from build123d import *

# Parameters (mm, degrees)
SKETCH1_R               = 32
BOSS_EXTRUDE1_DEPTH     = 15
SKETCH2_R               = 7
SKETCH2_R_2             = 6.446135322
BOSS_EXTRUDE2_DEPTH     = 15
SKETCH3_R               = 5.5
BOSS_EXTRUDE3_DEPTH     = 79
CUT_EXTRUDE1_DEPTH      = 79
CUT_EXTRUDE1_DEPTH_BACK = 79


with BuildPart() as part:
    # Sketch1 → Boss-Extrude1 (new body)
    with BuildSketch(Plane(origin=(0, 0, 0), x_dir=(1, 0, 0), z_dir=(0, 1, 0))):
        Circle(SKETCH1_R)
    extrude(amount=BOSS_EXTRUDE1_DEPTH)

    # Sketch2 → Boss-Extrude2 (add)
    with BuildSketch(Plane(origin=(0, 15, 0), x_dir=(1, 0, 0), z_dir=(0, 1, 0))):
        with Locations((25, 0)):
            Circle(SKETCH2_R)
        with Locations((-13, 22)):
            Circle(SKETCH2_R_2)
        with Locations((-13, -22)):
            Circle(SKETCH2_R_2)
    extrude(amount=BOSS_EXTRUDE2_DEPTH)

    # Sketch3 → Boss-Extrude3 (add)
    with BuildSketch(Plane(origin=(0, 15, 0), x_dir=(1, 0, 0), z_dir=(0, 1, 0))):
        Circle(SKETCH3_R)
    extrude(amount=BOSS_EXTRUDE3_DEPTH)

    # Sketch4 → Cut-Extrude1 (cut, two sides)
    with BuildSketch(Plane(origin=(0, 0, 0), x_dir=(0, 0, -1), z_dir=(1, 0, 0))) as cut_extrude1_sk:
        Polygon((-4.5, 84), (-8.757640736, 84), (-8.757640736, 94), (-4.5, 94), (-4, 94), (-4, 84), align=None)
    extrude(amount=CUT_EXTRUDE1_DEPTH, mode=Mode.SUBTRACT)
    extrude(cut_extrude1_sk.sketch, amount=-CUT_EXTRUDE1_DEPTH_BACK, mode=Mode.SUBTRACT)


solid = part.part
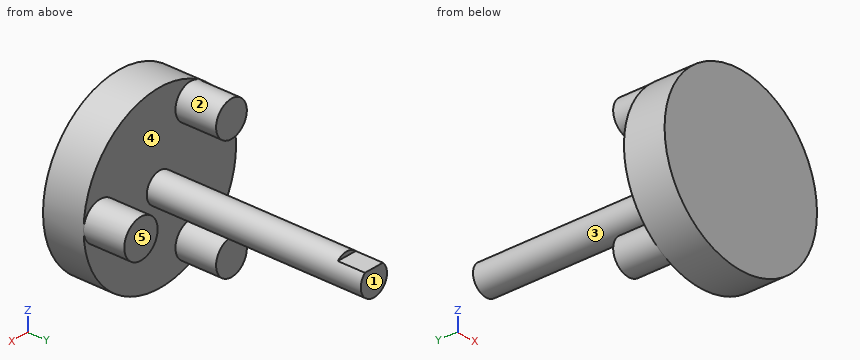
Geometry: final body of the model. Coordinates: model frame, mm. Face numbers are marked on the shaded views. A direction names the side the tool comes from. Round coordinates to 2 decimals unless told otherwise and drop trailing zeros. Order: outer loops, then holes, each group sorted by start corner. A loop starts at its lowest first (then second) coordinate and runs counter-clockwise, first axis right, second up. Notation, with made-up numbers: (51, -7.75) - (79, -7.75) arc R29 cw to (79, 21.25) - close; hole circle Ø1 at (-16, -12.5). An arc over 180 degrees is marked (long way). Write each question's results on one line, items separated by ' | '.
Item 1: Section C-C, the plane y = 45. Return the cut outline in (x, z).
Completed:
outline: circle Ø11 at (0, 0)
Item 2: Mould query, pull axis Z, two halves, no side actions, for the marked faces 3, 4 and 5. Classes: pulls with the +Z half, pulls with the -Z half, needs draft (parallel to the pull), parting line crosses it, or undercut.
Completed:
face 3: parting line crosses it | face 4: undercut | face 5: needs draft
Item 3: Section A-A, the plane x = 0. Return the cut outline in (y, z), and give its area (3 significant figures).
Completed:
outline: (0, -32) - (15, -32) - (15, -5.5) - (94, -5.5) - (94, 4) - (84, 4) - (84, 5.5) - (15, 5.5) - (15, 32) - (0, 32) - close | area: 1,810 mm^2
Item 4: Material intervals for line 1 along Y through (x, z) = (-6, 26); line 2 along Z through (x, y) = (23, 21); line 3 along Z through (x, y) = (-3.5, 89), sorted ascending. Write a range as [from, to].
Completed:
line 1: [0, 15] | line 2: [-6.71, 6.71] | line 3: [-4.24, 4]
Item 5: Section B-B, the plane z = -4. Return the cut outline in (x, y), and give its area (3 significant figures).
Completed:
outline: (-31.75, 0) - (31.75, 0) - (31.75, 15) - (30.74, 15) - (30.74, 30) - (19.26, 30) - (19.26, 15) - (3.77, 15) - (3.77, 94) - (-3.77, 94) - (-3.77, 15) - (-31.75, 15) - close | area: 1,720 mm^2
Item 6: Section D-D, the plane z = -25. Return the cut outline in (x, y).
Completed:
outline: (-19.97, 0) - (19.97, 0) - (19.97, 15) - (-7.29, 15) - (-7.29, 30) - (-18.71, 30) - (-18.71, 15) - (-19.97, 15) - close
Item 7: Reachability of the marked faces 1 and 2 from +Z, -Z, +X, -X, +Y, -Y: full face, straight path, thin tool, end or side. Return the list, or none.
Completed:
face 1: +Z, -Z, +X, -X, +Y | face 2: +Y
Item 8: First-contact query: pin 1 Ø4 at (x, z) = (-12, 25) entering from +Y; pin 2 Ø0.8 at (x, z) = (2, 4.5) entering from +Y; pin 3 Ø5 at (y, z) = (50.5, 9) entering from -X; pin 4 Ø4 at (x, y) = (1, 88) entering from +Z. Flat tips, straight axial feed; report the tip coordinate or a pass-through.
Completed:
pin 1: y = 30 | pin 2: y = 84 | pin 3: through | pin 4: z = 4
